Geometry: final body of the model. Coordinates: model frame, mm. A direction names the side the tool comes from. Round coordinates to 2 decimals unless told otherwise and drop trailing zeros. Write each loop counter-clockwise with the first axis right and the second up, starting at its lowest first coordinate (ties: lowest second). Pieces come first, ordered by that corner, then holes. Notation, with made-up numbers: M 14.5,87.5 L 47.5,87.5 A28 cw 47.5,116.5 Z; hole C 7,-10 d3. An arc over 180 degrees is marked long. Answer as CSV lines item,"result". Start each with the question number.
Q1. Section query B-B on x = 0. Output: boundary loops of the cut face in (y, z) (3 decimals).
Q2. Ray query, probe 1 along X at (y, z) = (1.3, -31.75); probe 2 along Z at (x, y) = (-44.45, 2.4); probe 3 along X at (y, z) = (0.6, 28). Return the intervals inside material, ascending.
Q3. Section query C-C on y = 1.5. Give the number of separate pieces and of enclosed holes in the cut face, and give its area (3 significant figures).
Q4. Mould query, pull axis Z, two halves, no side actions, for faces 1 (the cylindrical face through (48.89, 1.61, 36.29)), 2 (the flat face through (-6.35, 2, -28)), 3 (the flat face through (50.8, 2, 0)), 4 (the flat face through (41.91, 2, 0)). Classes: pulls with the +Z half, pulls with the -Z half, needs draft (parallel to the pull), parting line crosses it, or undercut.
Q5. First-contact query: pin 1 (2.5 mm diameter, centred on x = -44.45, z = -31.75, fed in from -Y). Flat tip, straight axial feed; report the tip coordinate or a pass-through.
Q6. Reachability of faces 5 (the flat face through (-40, 2, -6.35)), 6 (the flat face through (-1, 2, 38.1)) from +Z, -Z, +X, -X, +Y, -Y: full face, straight path, thin tool, end or side. Return the list, or none.
Q7. Section query A-A on z = 0. Output: boundary loops of the cut face in (x, y) (3 decimals), and give its area (3 significant figures).
```python
from build123d import *

# Parameters (mm, degrees)
SKETCH1_W           = 101.6
SKETCH1_H           = 76.2
BOSS_EXTRUDE1_DEPTH = 3.175
FILLET1_R           = 6.35
SKETCH2_R           = 2.2479
CUT_EXTRUDE1_DEPTH  = 4.175
SKETCH3_R           = 8.255
SKETCH3_R_2         = 1.2192
CUT_EXTRUDE2_DEPTH  = 4.175


with BuildPart() as part:
    # Sketch1 → Boss-Extrude1 (new body)
    with BuildSketch(Plane(origin=(0, 0, 0), x_dir=(1, 0, 0), z_dir=(0, 1, 0))):
        Rectangle(SKETCH1_W, SKETCH1_H)
    extrude(amount=BOSS_EXTRUDE1_DEPTH)

    # Fillet1
    fillet1_edges = [part.edges().sort_by_distance(p)[0] for p in [
        (50.8, 1.5875, 38.1),
        (-50.8, 1.5875, 38.1),
        (-50.8, 1.5875, -38.1),
        (50.8, 1.5875, -38.1),
    ]]
    fillet(fillet1_edges, radius=FILLET1_R)

    # Sketch2 → Cut-Extrude1 (cut, through all)
    with BuildSketch(Plane(origin=(0, 3.175, 0), x_dir=(1, 0, 0), z_dir=(0, 1, 0))):
        with Locations((-44.45, 31.75)):
            Circle(SKETCH2_R)
        with Locations((44.45, 31.75)):
            Circle(SKETCH2_R)
        with Locations((44.45, -31.75)):
            Circle(SKETCH2_R)
        with Locations((-44.45, -31.75)):
            Circle(SKETCH2_R)
        Polygon((-41.91, 0), (-41.91, 6.35), (-38.735, 6.35), (-38.735, -6.35), (-41.91, -6.35), align=None)
        Polygon((0, 29.21), (6.35, 29.21), (6.35, 26.035), (-6.35, 26.035), (-6.35, 29.21), align=None)
        Polygon((41.91, 0), (41.91, 6.35), (38.735, 6.35), (38.735, -6.35), (41.91, -6.35), align=None)
        Polygon((0, -29.21), (6.35, -29.21), (6.35, -26.035), (-6.35, -26.035), (-6.35, -29.21), align=None)
    extrude(amount=-CUT_EXTRUDE1_DEPTH, mode=Mode.SUBTRACT)

    # Sketch3 → Cut-Extrude2 (cut, through all)
    with BuildSketch(Plane(origin=(0, 3.175, 0), x_dir=(1, 0, 0), z_dir=(0, 1, 0))):
        Circle(SKETCH3_R)
        with Locations((-8.6995, -6.1341)):
            Circle(SKETCH3_R_2)
        with Locations((8.6995, 6.1341)):
            Circle(SKETCH3_R_2)
    extrude(amount=-CUT_EXTRUDE2_DEPTH, mode=Mode.SUBTRACT)


solid = part.part
```
Entries:
1,outline,"M 0,-38.1 L 3.175,-38.1 L 3.175,-29.21 L 0,-29.21 Z; M 0,-26.035 L 3.175,-26.035 L 3.175,-8.255 L 0,-8.255 Z; M 0,8.255 L 3.175,8.255 L 3.175,26.035 L 0,26.035 Z; M 0,29.21 L 3.175,29.21 L 3.175,38.1 L 0,38.1 Z"
2,probe 1,"x = -50.8 to -46.7, -42.2 to 42.2, 46.7 to 50.8"
2,probe 2,"z = -38.1 to -34, -29.5 to 29.5, 34 to 38.1"
2,probe 3,"x = -50.8 to -6.35, 6.35 to 50.8"
3,separate pieces,"1"
3,enclosed holes,"11"
3,area,"7,260 mm^2"
4,face 1,"pulls with the +Z half"
4,face 2,"undercut"
4,face 3,"needs draft"
4,face 4,"undercut"
5,pin 1,"passes through"
6,face 5,"+Y, -Y"
6,face 6,"+Z, +X, -X, +Y, -Y"
7,outline,"M -50.8,0 L -41.91,0 L -41.91,3.175 L -50.8,3.175 Z; M -38.735,0 L -8.255,0 L -8.255,3.175 L -38.735,3.175 Z; M 8.255,0 L 38.735,0 L 38.735,3.175 L 8.255,3.175 Z; M 41.91,0 L 50.8,0 L 50.8,3.175 L 41.91,3.175 Z"
7,area,"250 mm^2"
